Could you check a few things on this model? Use its own coordinates, in mm. A direction names the side the tool comes from. Give positions to 0.01 mm unless a question says otherwise; leave off trailing zeros. Loops run counter-clockwise (first coordinate to the right, second up) from the corner with the lowest first, then second, coordinate; pieces in that order, holes last. Notation, with made-up numbers: M -39.5,-32.75 L -26.5,-32.75 A16 cw -26.5,-21.75 Z; hole C -14.5,30.5 d4. An arc over 180 degrees is marked long. Return JSON: item names as keys, results as strings. Group by question number.
1. For faces 1 (the cylindrical face through (-224.297, 57.594, -101.242)), 2 (the flat face through (-143, 98, -32)), 3 (the cylindrical face through (-224, 138.7, 39.3)), which set-ups out of +Z, -Z, +X, -X, +Y, -Y let a thin tool reach every point of the face, with its end or its side?
2. If we section it at D-D (y = 156.5): Write out the boundary of the cut face in (x, z).
3. If we section it at A-A (x = 87.5): Write out the boundary of the cut face in (y, z).
4. If we section it at C-C (z = 54): Write out the boundary of the cut face in (x, y).
5. If we mould it in two halves opening along X, with no side actions, what happens to faces 4 (the cylindrical face through (3.35, 193.52, 134.19)), 5 (the cylindrical face through (-148.703, 138.58, 39.029)), 6 (the flat face through (-55, 105, -18)), 7 (the flat face through (-70.867, 77.346, -65.06))? For each: +X half, -X half, draft (parallel to the pull), parting line (faces both ways), or undercut.
6. Please list where these lines run through material, in increasing order: line 1 (Z direction, x = -269.5, y = 169.5); line 2 (Z direction, x = 192.5, y = 37); line 3 (Y direction, x = -218.5, z = -105).
7. For pin 1 (8 mm diameter, centred on x = -143, y = 82, fed in from +Z); pin 2 (2 mm diameter, centred on x = -112.5, z = -46.5, fed in from +Y); pin 3 (20.5 mm diameter, centred on y = 85, z = -42.5, fed in from +X), each with a flat end and sliding along its axis, tell me the tip position at first contact or that it passes through.
8. If we section it at B-B (z = -69): Write out the boundary of the cut face in (x, y).
```python
from build123d import *

# Parameters (mm, degrees)
PAD003_DEPTH            = 2
SKETCH056_R             = 1.5
POCKET034_DEPTH         = 5
SKETCH063_R             = 1.5
POCKET039_DEPTH         = 5
BODY002_PLACEMENT_ANGLE = 330


with BuildPart() as part:
    # Sketch009 → Pad003 (new body)
    with BuildSketch(Plane.XZ):
        with BuildLine():
            Line((-300, -200), (300, -200))
            Line((300, -200), (300, -120))
            Line((-55, -120), (300, -120))
            Line((-55, 142), (-55, -120))
            Line((300, 142), (-55, 142))
            Line((300, 142), (300, 200))
            ThreePointArc((300, 200), (-0.8504900273, 188.6850121637), (-300, 154.7937598629))
            Line((-300, 154.7937598629), (-300, -200))
        make_face()
        with BuildLine():
            Line((-230, 65.1307599432), (-230, -68.8692400568))
            ThreePointArc((-230, -68.8692400568), (-224.1421356237, -83.0113756806), (-210, -88.8692400568))
            Line((-210, -88.8692400568), (-163, -88.8692400568))
            ThreePointArc((-163, -88.8692400568), (-148.8578643763, -83.0113756806), (-143, -68.8692400568))
            Line((-143, -68.8692400568), (-143, 65.1307599432))
            ThreePointArc((-143, 65.1307599432), (-148.8578643763, 79.2728955669), (-163, 85.1307599432))
            Line((-163, 85.1307599432), (-210, 85.1307599432))
            ThreePointArc((-210, 85.1307599432), (-224.1421356237, 79.2728955669), (-230, 65.1307599432))
        make_face(mode=Mode.SUBTRACT)
    extrude(amount=-PAD003_DEPTH)

    # Sketch056 (on Face2 of Binder014) → Pocket034 (cut)
    with BuildSketch(Plane(origin=(0, 3.7320508076, 0), x_dir=(-1, 0, 0), z_dir=(0, 1, 0))):
        with Locations((290, -190)):
            Circle(SKETCH056_R)
        with Locations((110, -190)):
            Circle(SKETCH056_R)
        with Locations((110, -100.851579)):
            Circle(SKETCH056_R)
        with Locations((110, -11.703157)):
            Circle(SKETCH056_R)
        with Locations((110, 82.445264)):
            Circle(SKETCH056_R)
        with Locations((110, 166.593685)):
            Circle(SKETCH056_R)
        with Locations((290, 143.673156)):
            Circle(SKETCH056_R)
        with Locations((290, 65.254867)):
            Circle(SKETCH056_R)
        with Locations((290, -23.163422)):
            Circle(SKETCH056_R)
        with Locations((290, -106.581711)):
            Circle(SKETCH056_R)
    extrude(amount=-POCKET034_DEPTH, mode=Mode.SUBTRACT)

    # Sketch063 (on Face5 of Pocket034) → Pocket039 (cut)
    with BuildSketch(Plane(origin=(0, 2, 0), x_dir=(1, 0, 0), z_dir=(0, 1, 0))):
        with Locations((-132, 190)):
            Circle(SKETCH063_R)
        with Locations((-200, 190)):
            Circle(SKETCH063_R)
        with Locations((-268, 190)):
            Circle(SKETCH063_R)
    extrude(amount=-POCKET039_DEPTH, mode=Mode.SUBTRACT)


with BuildPart() as part_1:
    # Body002 placement: moved
    add(part.part.moved(Location((0, 98.1679491924, -28.9949192431))).rotate(Axis((0, 98.1679491924, -28.9949192431), (1, 0, 0)), BODY002_PLACEMENT_ANGLE))


solid = part_1.part
```
Answer:
{
 "1": {"face 1": "+Z, +Y", "face 2": "+Z, -Z, +Y, -Y", "face 3": "-Z, -Y"},
 "2": {"outline": "M -300,68.04 L -55,68.04 L -55,72.04 L -300,72.04 Z"},
 "3": {"outline": "M -1.83,-202.2 L -0.1,-203.2 L 39.9,-133.92 L 38.17,-132.92 Z; M 169.17,93.98 L 170.9,92.98 L 197.08,138.33 L 195.35,139.33 Z"},
 "4": {"outline": "M -300,146.09 L -55,146.09 L -55,148.39 L -300,148.39 Z"},
 "5": {"face 4": "-X half", "face 5": "undercut", "face 6": "+X half", "face 7": "draft"},
 "6": {"line 1": "z = 90.56 to 94.56", "line 2": "z = -138.94 to -134.94", "line 3": "y = 54.29 to 55.87"},
 "7": {"pin 1": "stops at z = -50.07", "pin 2": "stops at y = 90.95", "pin 3": "stops at x = -55"},
 "8": {"outline": "M -300,75.07 L -230,75.07 L -230,77.38 L -300,77.38 Z; M -143,75.07 L -55,75.07 L -55,77.38 L -143,77.38 Z"}
}
